The model under review builds one solid part; all positions refer to its coordinate system, in mm. Face numbers are marked on the shaded views. A direction names the side the tool comes from. Round coordinates to 2 decimals unless told otherwise and drop trailing zeros. Order: outer loops, then holes, each group sorted by start corner. A loop starts at its lowest first (then second) coordinate and runs counter-clockwise, first axis right, second up. Notation, with made-up numbers: M 86,-29.75 L 111,-29.75 A21 cw 111,-11.75 Z; hole C 3,-35 d10. An arc over 180 degrees is marked long. Answer as a JSON object with one key per item and string values. Group by question number.
1) Consider section A-A, the plane y = 7.25. Write out the cut boundary in (x, z), then the cut area to 3 significant figures.
2) Consider section C-C, the plane z = 3. Write out the cut boundary in (x, y), then the cut area to 3 significant figures.
3) Consider section D-D, the plane z = 14. Write out the cut boundary in (x, y), then the cut area to 3 significant figures.
4) To check wall thickness, follow line 1 (X direction, y = 5, z = 4.5); line 2 (Z direction, x = 36, y = 5.75); line 3 (X direction, y = 7.5, z = 20). State the ranges of each line that lie inside material, in increasing order.
5) The part is to be moulded in two halves that separate along Z. For the marked faces 3, 4 and 5, say which applies: +Z half, -Z half, draft (parallel to the pull), parting line (faces both ways), or undercut.
6) Consider section B-B, the plane x = 16.5. Write out the cut boundary in (y, z).
7) Insertion check: pin 1 Ø2 at (x, z) = (6, 6) entering from +Y; pin 2 Ø2.5 at (y, z) = (4.5, 6) entering from +X; pin 3 Ø5 at (y, z) = (7, 27) entering from -X. Each pin has a flat end and moves straight along its axis. Give the tip position at first contact, or say it passes through.
8) For the marked faces 1 and 2, list the 3-axis set-ups (+Z, -Z, +X, -X, +Y, -Y) from which the entire face can be reached by the end or side of a thin tool; tool diameter is ignored.
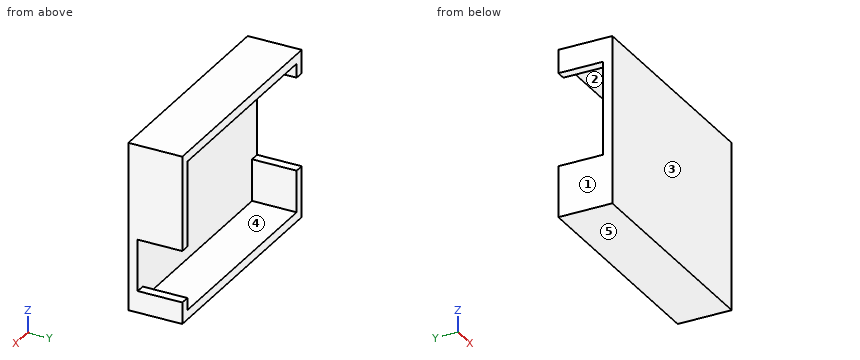
```python
from build123d import *

# Parameters (mm, degrees)
ESQUISSE1_W        = 47.5
ESQUISSE1_H        = 35.8
BOSS_EXTRU_2_DEPTH = 2
ESQUISSE2_W        = 47.5
ESQUISSE2_H        = 2
BOSS_EXTRU_3_DEPTH = 9.5
ESQUISSE3_W        = 47.5
ESQUISSE3_H        = 2
BOSS_EXTRU_4_DEPTH = 9.5
ESQUISSE4_W        = 2
ESQUISSE4_H        = 2.6
BOSS_EXTRU_5_DEPTH = 9.5
ESQUISSE5_W        = 2
ESQUISSE5_H        = 18.2
BOSS_EXTRU_6_DEPTH = 9.5
ESQUISSE6_W        = 2
ESQUISSE6_H        = 8.9
BOSS_EXTRU_7_DEPTH = 9.5
ESQUISSE8_W        = 2
ESQUISSE8_H        = 3
BOSS_EXTRU_8_DEPTH = 9.5


with BuildPart() as part:
    # Esquisse1 → Boss.-Extru.2 (new body)
    with BuildSketch(Plane(origin=(0, 0, 0), x_dir=(1, 0, 0), z_dir=(0, 1, 0))):
        with Locations((23.75, -17.9)):
            Rectangle(ESQUISSE1_W, ESQUISSE1_H)
    extrude(amount=BOSS_EXTRU_2_DEPTH)

    # Esquisse2 → Boss.-Extru.3 (add)
    with BuildSketch(Plane(origin=(0, 2, 0), x_dir=(1, 0, 0), z_dir=(0, 1, 0))):
        with Locations((23.75, -34.8)):
            Rectangle(ESQUISSE2_W, ESQUISSE2_H)
    extrude(amount=BOSS_EXTRU_3_DEPTH)

    # Esquisse3 → Boss.-Extru.4 (add)
    with BuildSketch(Plane(origin=(0, 2, 0), x_dir=(1, 0, 0), z_dir=(0, 1, 0))):
        with Locations((23.75, -1)):
            Rectangle(ESQUISSE3_W, ESQUISSE3_H)
    extrude(amount=BOSS_EXTRU_4_DEPTH)

    # Esquisse4 → Boss.-Extru.5 (add)
    with BuildSketch(Plane(origin=(0, 2, 0), x_dir=(1, 0, 0), z_dir=(0, 1, 0))):
        with Locations((46.5, -3.3)):
            Rectangle(ESQUISSE4_W, ESQUISSE4_H)
    extrude(amount=BOSS_EXTRU_5_DEPTH)

    # Esquisse5 → Boss.-Extru.6 (add)
    with BuildSketch(Plane(origin=(0, 2, 0), x_dir=(1, 0, 0), z_dir=(0, 1, 0))):
        with Locations((46.5, -24.7)):
            Rectangle(ESQUISSE5_W, ESQUISSE5_H)
    extrude(amount=BOSS_EXTRU_6_DEPTH)

    # Esquisse6 → Boss.-Extru.7 (add)
    with BuildSketch(Plane(origin=(0, 2, 0), x_dir=(1, 0, 0), z_dir=(0, 1, 0))):
        with Locations((1, -6.45)):
            Rectangle(ESQUISSE6_W, ESQUISSE6_H)
    extrude(amount=BOSS_EXTRU_7_DEPTH)

    # Esquisse8 → Boss.-Extru.8 (add)
    with BuildSketch(Plane(origin=(0, 2, 0), x_dir=(1, 0, 0), z_dir=(0, 1, 0))):
        with Locations((1, -32.3)):
            Rectangle(ESQUISSE8_W, ESQUISSE8_H)
    extrude(amount=BOSS_EXTRU_8_DEPTH)


solid = part.part
```
Results list:
{
 "1": {"outline": "M 0,0 L 47.5,0 L 47.5,4.6 L 45.5,4.6 L 45.5,2 L 2,2 L 2,10.9 L 0,10.9 Z; M 0,30.8 L 2,30.8 L 2,33.8 L 45.5,33.8 L 45.5,15.6 L 47.5,15.6 L 47.5,35.8 L 0,35.8 Z", "area": "255 mm^2"},
 "2": {"outline": "M 0,0 L 47.5,0 L 47.5,11.5 L 45.5,11.5 L 45.5,2 L 2,2 L 2,11.5 L 0,11.5 Z", "area": "133 mm^2"},
 "3": {"outline": "M 0,0 L 47.5,0 L 47.5,2 L 0,2 Z", "area": "95.0 mm^2"},
 "4": {"line 1": "0 to 2, 45.5 to 47.5", "line 2": "0 to 2, 33.8 to 35.8", "line 3": "45.5 to 47.5"},
 "5": {"face 3": "draft", "face 4": "undercut", "face 5": "-Z half"},
 "6": {"outline": "M 0,0 L 11.5,0 L 11.5,2 L 2,2 L 2,33.8 L 11.5,33.8 L 11.5,35.8 L 0,35.8 Z"},
 "7": {"pin 1": "y = 2", "pin 2": "x = 2", "pin 3": "x = 45.5"},
 "8": {"face 1": "+Z, -Z, -X, +Y, -Y", "face 2": "+Y"}
}
